CAD build for the part. Positions are in the model's coordinates, mm. A direction names the side the tool comes from. Round coordinates to 2 decimals unless told otherwise and drop trailing zeros. Loops run counter-clockwise (first coordinate to the right, second up) from the corner with the lowest first, then second, coordinate; pieces in that order, holes last.
from build123d import *

# Parameters (mm, degrees)
SKETCH_R     = 4.76
PAD_DEPTH    = 6.35
SKETCH001_R  = 6.35
PAD001_DEPTH = 26.2
SKETCH002_R  = 1
PAD002_DEPTH = 5.8
SKETCH003_R  = 2.5
PAD003_DEPTH = 6
PAD004_DEPTH = 2
FILLET_R     = 1


with BuildPart() as part:
    # Sketch → Pad (new body)
    with BuildSketch(Plane.XY):
        Circle(SKETCH_R)
    extrude(amount=PAD_DEPTH)

    # Sketch001 (on Face3 of Pad) → Pad001 (join)
    with BuildSketch(Plane.XY.offset(6.35)):
        Circle(SKETCH001_R)
    extrude(amount=PAD001_DEPTH)

    # Sketch002 (on Face5 of Pad001) → Pad002 (join)
    with BuildSketch(Plane(origin=(0, 0, 0), x_dir=(1, 0, 0), z_dir=(0, 0, -1))):
        Circle(SKETCH002_R)
    extrude(amount=PAD002_DEPTH)

    # Sketch003 (on Face3 of Pad002) → Pad003 (join)
    with BuildSketch(Plane.XY.offset(32.55)):
        Circle(SKETCH003_R)
    extrude(amount=PAD003_DEPTH)

    # Sketch004 (on Face3 of Pad003) → Pad004 (join)
    with BuildSketch(Plane.XY.offset(32.55)):
        with BuildLine():
            ThreePointArc((1.736759, 5.586248), (0, 5.85), (-1.736759, 5.586248))
            Line((-1.736759, 4.421105), (-1.736759, 5.586248))
            ThreePointArc((1.736759, 4.421105), (0, 4.75), (-1.736759, 4.421105))
            Line((1.736759, 5.586248), (1.736759, 4.421105))
        make_face()
    extrude(amount=PAD004_DEPTH)

    # Fillet
    fillet_edges = [part.edges().sort_by_distance(p)[0] for p in [
        (-6.35, 0, 32.55),
    ]]
    fillet(fillet_edges, radius=FILLET_R)


solid = part.part
Item 1: Cut at C-C (z = 36). List the corners of the cut face in (x, y), plus the area to 3 significant figures.
Verdict:
outline: circle Ø5 at (0, 0)
area: 19.6 mm2
Item 2: Cut at B-B (z = 16). List the corners of the cut face in (x, y).
Verdict:
outline: circle Ø12.7 at (0, 0)
Item 3: 3-axis set-ups, long thin cutter, end or side, ignore diameter. For faces 1 (the flat face through (-1, -5, 6.35)), 2 (the flat face through (-1.737, 5, 34)), 3 (the cylindrical face through (0.02, 5.85, 33.54)), 4 (the flat face through (0, 5, 34.55)), 5 (the cylindrical face through (-0.54, -2.44, 35.51)): which of +Z, -Z, +X, -X, +Y, -Y reach the whole face in a straight line?
Verdict:
face 1: -Z
face 2: +Z, -X, +Y
face 3: +Z, +Y
face 4: +Z, +X, -X, +Y
face 5: +Z
Item 4: Flat gauge pins, fed straight in: P1, Ø3, axis at y = -4, z = 6, coming from the +X side; P2, Ø1.6, axis at x = 0.5, y = 5.5, coming from the +Z side; P3, Ø3, axis at x = 3, y = -4, coming from the +Z side. Where does each tip first touch, or does it go through?
Verdict:
P1: stops at x = 5.82
P2: stops at z = 34.55
P3: stops at z = 32.55
Item 5: Mould opens along Y. For faces 6 (the flat face through (1.737, 5, 34)), 7 (the cylindrical face through (-1.032, -4.647, 3.131)), 8 (the cylindrical face through (0.02, 4.75, 33.54)) say: released by +Y, released by -Y, zero draft, split by the parting line, or undercut.
Verdict:
face 6: zero draft
face 7: split by the parting line
face 8: undercut
Item 6: Cut at A-A (y = 0). List the corners of the cut face in (x, z).
Verdict:
outline: (-6.35, 6.35) - (-4.76, 6.35) - (-4.76, 0) - (-1, 0) - (-1, -5.8) - (1, -5.8) - (1, 0) - (4.76, 0) - (4.76, 6.35) - (6.35, 6.35) - (6.35, 31.55) arc R1 ccw to (5.35, 32.55) - (2.5, 32.55) - (2.5, 38.55) - (-2.5, 38.55) - (-2.5, 32.55) - (-5.35, 32.55) arc R1 ccw to (-6.35, 31.55) - close
Item 7: Wall check: L1, parallel to Z at x = 0.5, y = -5; L2, parallel to Z at x = -1, y = 5; L3, parallel to X at y = -0.25, z = 5. Give the ranges that are in metal, low to high.
Verdict:
L1: z = 6.35 to 32.55
L2: z = 6.35 to 34.55
L3: x = -4.75 to 4.75
